CAD build for the part. Positions are in the model's coordinates, mm. A direction names the side the tool comes from. Give positions to 0.01 mm unless a question says otherwise; leave off trailing zeros. Loops run counter-clockwise (first coordinate to the right, second up) from the corner with the lowest first, then second, coordinate; pieces in that order, holes last. Notation, with made-up numbers: M 64,-10 L 119,-10 A30 ccw 119,13 Z; hole C 48,-31 d6. An arc over 180 degrees is marked long. Answer as CSV lines item,"result".
from build123d import *

# Parameters (mm, degrees)
SKETCH_1_R          = 1.6
EXTRUDE_1_DEPTH     = 16
CUT_EXTRUDE_1_REACH = 64.298
SKETCH_2_R          = 1.6
CUT_EXTRUDE_2_REACH = 64.298
SKETCH_3_R          = 1.6


with BuildPart() as part:
    # 草图1 → 凸台-拉伸1 (new body)
    with BuildSketch(Plane(origin=(0, 0, 0), x_dir=(1, 0, 0), z_dir=(0, 1, 0))):
        Polygon((0, 0), (32, 0), (32, -18), (12, -18), (12, -33), (32, -33), (32, -51), (0, -51), align=None)
        with Locations(Location((19.5, -13, 0), (0, 0, 270))):
            Circle(SKETCH_1_R, mode=Mode.SUBTRACT)
        with Locations(Location((19.5, -5, 0), (0, 0, 270))):
            Circle(SKETCH_1_R, mode=Mode.SUBTRACT)
        with Locations(Location((27.5, -5, 0), (0, 0, 270))):
            Circle(SKETCH_1_R, mode=Mode.SUBTRACT)
        with Locations(Location((27.5, -13, 0), (0, 0, 270))):
            Circle(SKETCH_1_R, mode=Mode.SUBTRACT)
        with Locations(Location((11.5, -5, 0), (0, 0, 270))):
            Circle(SKETCH_1_R, mode=Mode.SUBTRACT)
        with Locations(Location((11.5, -13, 0), (0, 0, 270))):
            Circle(SKETCH_1_R, mode=Mode.SUBTRACT)
        with Locations(Location((27.5, -38, 0), (0, 0, 90))):
            Circle(SKETCH_1_R, mode=Mode.SUBTRACT)
        with Locations(Location((19.5, -38, 0), (0, 0, 90))):
            Circle(SKETCH_1_R, mode=Mode.SUBTRACT)
        with Locations(Location((11.5, -38, 0), (0, 0, 90))):
            Circle(SKETCH_1_R, mode=Mode.SUBTRACT)
        with Locations(Location((27.5, -46, 0), (0, 0, 90))):
            Circle(SKETCH_1_R, mode=Mode.SUBTRACT)
        with Locations(Location((19.5, -46, 0), (0, 0, 90))):
            Circle(SKETCH_1_R, mode=Mode.SUBTRACT)
        with Locations(Location((11.5, -46, 0), (0, 0, 90))):
            Circle(SKETCH_1_R, mode=Mode.SUBTRACT)
        with Locations(Location((7, -25.5, 0), (0, 0, 270))):
            Circle(SKETCH_1_R, mode=Mode.SUBTRACT)
    extrude(amount=EXTRUDE_1_DEPTH)

    # 切除-拉伸1: up to this face of the body (flat: up to its plane)
    cut_extrude_1_end = Plane(part.part.faces().sort_by_distance((16, 8, 0))[0])
    # 草图2 → 切除-拉伸1 (cut, up to the picked face)
    with BuildSketch(Plane.XY.offset(51), mode=Mode.PRIVATE) as cut_extrude_1_sk1:
        with Locations((19.5, 12)):
            Circle(SKETCH_2_R)
    cut_extrude_1_tool1 = split(extrude(cut_extrude_1_sk1.sketch, amount=-CUT_EXTRUDE_1_REACH, mode=Mode.PRIVATE), bisect_by=cut_extrude_1_end, keep=Keep.BOTH, mode=Mode.PRIVATE)
    # 草图2 → 切除-拉伸1 (cut, up to the picked face)
    with BuildSketch(Plane.XY.offset(51), mode=Mode.PRIVATE) as cut_extrude_1_sk2:
        with Locations((19.5, 5)):
            Circle(SKETCH_2_R)
    cut_extrude_1_tool2 = split(extrude(cut_extrude_1_sk2.sketch, amount=-CUT_EXTRUDE_1_REACH, mode=Mode.PRIVATE), bisect_by=cut_extrude_1_end, keep=Keep.BOTH, mode=Mode.PRIVATE)
    add(cut_extrude_1_tool1.solids().sort_by(Axis((19.5, 12, 51), (0, 0, -1)))[0], mode=Mode.SUBTRACT)
    add(cut_extrude_1_tool2.solids().sort_by(Axis((19.5, 5, 51), (0, 0, -1)))[0], mode=Mode.SUBTRACT)

    # 切除-拉伸2: up to this face of the body (flat: up to its plane)
    cut_extrude_2_end = Plane(part.part.faces().sort_by_distance((12, 8, 25.5))[0])
    # 草图3 → 切除-拉伸2 (cut, up to the picked face)
    with BuildSketch(Plane.ZY, mode=Mode.PRIVATE) as cut_extrude_2_sk1:
        with Locations((25.5, 5)):
            Circle(SKETCH_3_R)
    cut_extrude_2_tool1 = split(extrude(cut_extrude_2_sk1.sketch, amount=-CUT_EXTRUDE_2_REACH, mode=Mode.PRIVATE), bisect_by=cut_extrude_2_end, keep=Keep.BOTH, mode=Mode.PRIVATE)
    # 草图3 → 切除-拉伸2 (cut, up to the picked face)
    with BuildSketch(Plane.ZY, mode=Mode.PRIVATE) as cut_extrude_2_sk2:
        with Locations((25.5, 12)):
            Circle(SKETCH_3_R)
    cut_extrude_2_tool2 = split(extrude(cut_extrude_2_sk2.sketch, amount=-CUT_EXTRUDE_2_REACH, mode=Mode.PRIVATE), bisect_by=cut_extrude_2_end, keep=Keep.BOTH, mode=Mode.PRIVATE)
    add(cut_extrude_2_tool1.solids().sort_by(Axis((0, 5, 25.5), (1, 0, 0)))[0], mode=Mode.SUBTRACT)
    add(cut_extrude_2_tool2.solids().sort_by(Axis((0, 12, 25.5), (1, 0, 0)))[0], mode=Mode.SUBTRACT)


solid = part.part
1) Band-saw the part on B-B on y = 2.5. Give the number of separate pieces and of enclosed holes in the cut face, and give its area (3 significant figures).
Answer below:
separate pieces,"1"
enclosed holes,"13"
area,"1,230 mm^2"
2) Flat gauge pins, fed straight in: pin 1 (4 mm diameter, centred on y = 12, z = 25.5, fed in from +X); pin 2 (6 mm diameter, centred on x = 21.5, z = 22.5, fed in from +Y). Where does each tip first touch, or does it go through?
Answer below:
pin 1,"stops at x = 12"
pin 2,"passes through"
3) Drill centre lines: line 1 (Z direction, x = 23.5, y = 9.5); line 2 (Z direction, x = 27, y = 11.5); line 3 (X direction, y = 1.65, z = 25.5). Where is each one in solid material? Low to high. Write a range as from..to.
Answer below:
line 1,"z = 0..18, 33..51"
line 2,"z = 0..3.48, 6.52..11.48, 14.52..18, 33..36.48, 39.52..44.48, 47.52..51"
line 3,"x = 0..5.4, 8.6..12"
4) Mould opens along Z. For faces 1 (the face through (2.67, 5.07, 23.9)), 2 (the face through (20.98, 4.39, 16.09)), 3 (the face through (16, 8, 0)) say: +Z half, -Z half, draft (parallel to the pull), parting line (faces both ways), or undercut.
Answer below:
face 1,"undercut"
face 2,"draft"
face 3,"-Z half"
5) Band-saw the part on D-D on x = 3.5. Give the cut face in (y, z), and give its area (3 significant figures).
Answer below:
outline,"M 0,0 L 16,0 L 16,51 L 0,51 Z; hole C 5,25.5 d3.2; hole C 12,25.5 d3.2"
area,"800 mm^2"
6) Band-saw the part on C-C on z = 25.5. Give the cut face in (x, y), and give its area (3 significant figures).
Answer below:
outline,"M 0,0 L 5.4,0 L 5.4,3.4 L 0,3.4 Z; M 0,6.6 L 5.4,6.6 L 5.4,10.4 L 0,10.4 Z; M 0,13.6 L 5.4,13.6 L 5.4,16 L 0,16 Z; M 8.6,0 L 12,0 L 12,3.4 L 8.6,3.4 Z; M 8.6,6.6 L 12,6.6 L 12,10.4 L 8.6,10.4 Z; M 8.6,13.6 L 12,13.6 L 12,16 L 8.6,16 Z"
area,"84.5 mm^2"
7) Band-saw the part on A-A on x = 27.5. Give the cut face in (y, z).
Answer below:
outline,"M 0,0 L 16,0 L 16,3.4 L 0,3.4 Z; M 0,6.6 L 16,6.6 L 16,11.4 L 0,11.4 Z; M 0,14.6 L 16,14.6 L 16,18 L 0,18 Z; M 0,33 L 16,33 L 16,36.4 L 0,36.4 Z; M 0,39.6 L 16,39.6 L 16,44.4 L 0,44.4 Z; M 0,47.6 L 16,47.6 L 16,51 L 0,51 Z"
8) Which spindle directions (+Z, -Z, +X, -X, +Y, -Y) get a long thin tool onto all of the face, cutting with end or side? Do faces 4 (the face through (12, 8, 25)), 5 (the face through (17.914, 1.909, 38.208)). Say none if no direction does.
Answer below:
face 4,"+X, +Y, -Y"
face 5,"+Y, -Y"
